Can you work these out from the drawing? Everything is in mm from the part's minimum corner. Give positions to 0.01 mm unless a question says otherwise; leave off trailing zeros. Loops run counter-clockwise (first coordinate to the right, second up) from the corner with the lowest first, then second, coordinate; pieces in that order, holes last. Notation, with made-up numbers: (31.5, 48.25) - (85.5, 48.25) arc R23 cw to (85.5, 61.25) - close; hole circle Ø3 at (70, -22). An arc over 180 degrees is marked (long way). Answer in a Markdown table with one row per item.
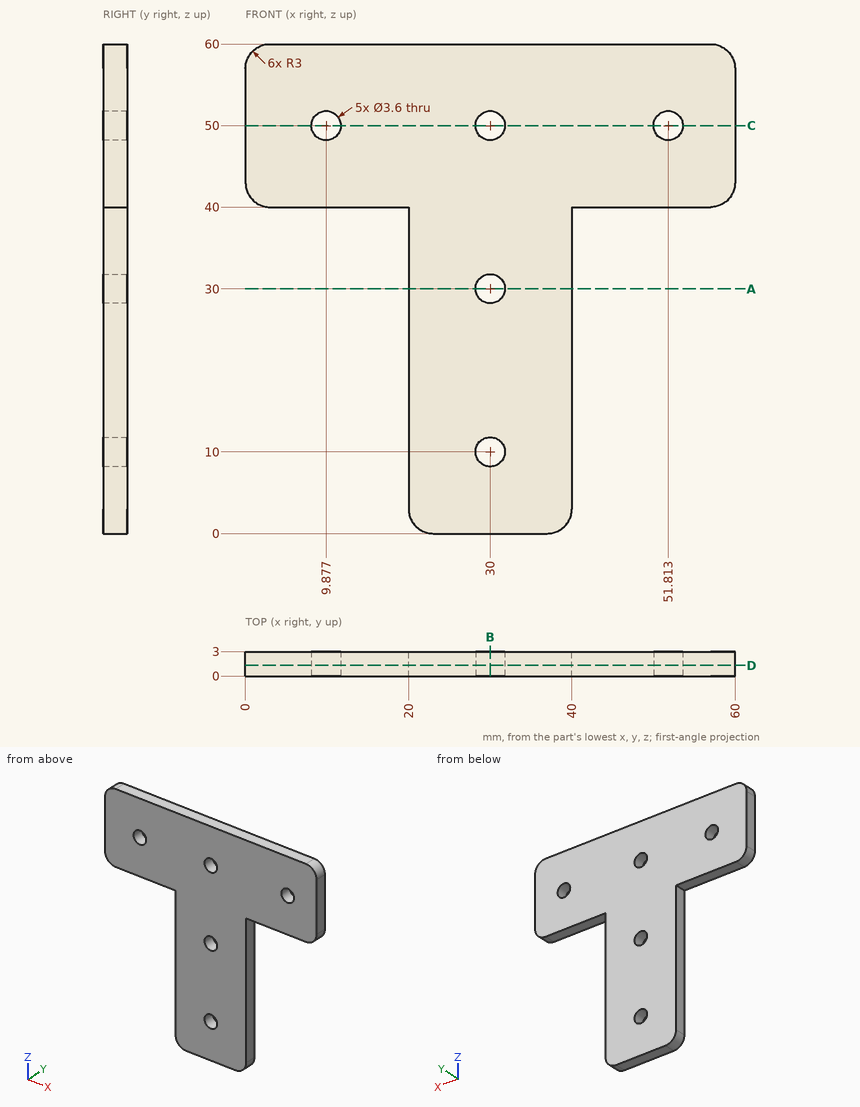
Q1. Imagine slicing it at C-C, the plane z = 50. Write out the boundary of the cut face in (x, y).
Checked values:
| item | result |
|---|---|
| outline | (0, 0) - (8.08, 0) - (8.08, 3) - (0, 3) - close; (11.68, 0) - (28.2, 0) - (28.2, 3) - (11.68, 3) - close; (31.8, 0) - (50.01, 0) - (50.01, 3) - (31.8, 3) - close; (53.61, 0) - (60, 0) - (60, 3) - (53.61, 3) - close |
Q2. Imagine slicing it at A-A, the plane z = 30. Write out the boundary of the cut face in (x, y).
Checked values:
| item | result |
|---|---|
| outline | (20, 0) - (28.2, 0) - (28.2, 3) - (20, 3) - close; (31.8, 0) - (40, 0) - (40, 3) - (31.8, 3) - close |
Q3. Imagine slicing it at B-B, the plane x = 30. Write out the boundary of the cut face in (y, z), and give its area (3 significant figures).
Checked values:
| item | result |
|---|---|
| outline | (0, 0) - (3, 0) - (3, 8.2) - (0, 8.2) - close; (0, 11.8) - (3, 11.8) - (3, 28.2) - (0, 28.2) - close; (0, 31.8) - (3, 31.8) - (3, 48.2) - (0, 48.2) - close; (0, 51.8) - (3, 51.8) - (3, 60) - (0, 60) - close |
| area | 148 mm² |
Q4. If I drill on line 1 (X direction, y = 1.45, z = 50); line 2 (X direction, y = 2.5, z = 10); line 3 (X direction, y = 2.3, z = 48.5) (1 decimal), over which ranges is the centre line in solid material (lowest first)? Write a range as [from, to].
Checked values:
| item | result |
|---|---|
| line 1 | x = [0, 8.08], [11.68, 28.2], [31.8, 50.01], [53.61, 60] |
| line 2 | x = [20, 28.2], [31.8, 40] |
| line 3 | x = [0, 8.9], [10.9, 29], [31, 50.8], [52.8, 60] |
Q5. Imagine slicing it at D-D, the plane y = 1.3. Write out the boundary of the cut face in (x, z), and give its area (3 significant figures).
Checked values:
| item | result |
|---|---|
| outline | (0, 43) arc R3 ccw to (3, 40) - (20, 40) - (20, 3) arc R3 ccw to (23, 0) - (37, 0) arc R3 ccw to (40, 3) - (40, 40) - (57, 40) arc R3 ccw to (60, 43) - (60, 57) arc R3 ccw to (57, 60) - (3, 60) arc R3 ccw to (0, 57) - close; hole circle Ø3.6 at (9.88, 50); hole circle Ø3.6 at (30, 10); hole circle Ø3.6 at (30, 30); hole circle Ø3.6 at (30, 50); hole circle Ø3.6 at (51.81, 50) |
| area | 1,940 mm² |
Q6. For pin 1 (3 mm diameter, centred on x = 30, z = 30, fed in from -Y); pin 2 (1.5 mm diameter, centred on y = 1, z = 16.5, fed in from +X); pin 3 (1.5 mm diameter, centred on x = 13.5, y = 2, fed in from -Z), each with a flat end and sliding along its axis, tell me the tip position at first contact or that it passes through.
Checked values:
| item | result |
|---|---|
| pin 1 | passes through |
| pin 2 | stops at x = 40 |
| pin 3 | stops at z = 40 |
